Could you check a few things on this model? Use its own coordinates, in mm. A direction names the side the tool comes from. Coordinates: 2 decimals unless noted, no trailing zeros. Order: outer loops, then holes, each group sorted by start corner. A loop starts at its lowest first (then second) coordinate and runs counter-clockwise, first axis right, second up. Notation, with made-up numbers: (76.25, -7) - (134.25, -7) arc R25 cw to (134.25, 28) - close; hole circle Ø10 at (59.25, 4). An arc over 180 degrees is marked (long way). Answer as a JSON object with one key per item and string values. Group by question number.
(1) Imagine slicing it at C-C, the plane z = 3.6. Give the number of separate pieces and of enclosed holes in the cut face, and give its area (3 significant figures).
(2) We'd pull the mould along Y, two halves only. Please class faces 1 (the cylindrical face through (109.745, -109.861, 2.958)), 2 (the flat face through (-2, 2, 6)), 3 (the flat face through (-5, 69, 3)): pulls with the +Y half, pulls with the -Y half, needs draft (parallel to the pull), parting line crosses it, or undercut.
(3) Which directions (+Z, -Z, +X, -X, +Y, -Y) give clear straight access to the entire face, cutting with the end or side of a thin tool? Please do faces 4 (the flat face through (112, -1, 3)), 5 (the cylindrical face through (73.877, 93.387, 2.958)).
(4) Imagine slicing it at A-A, the plane y = -6. Write out the boundary of the cut face in (x, z).
(5) Please list where these lines run through material, in increasing order: probe 1 along Y at (x, z) = (13.5, 2.4); probe 2 along Y at (x, z) = (-97.5, 3.75); probe 3 along X at (y, z) = (104.5, 1.45).
(6) Imagine slicing it at B-B, the plane x = 63. Write out the boundary of the cut face in (y, z), and give its area (3 significant figures).
from build123d import *

# Parameters (mm, degrees)
F0_R     = 1.5
F0_R_2   = 2.25
F1_DEPTH = 6


with BuildPart() as f1:
    # F0 (on Top) → F1 (new body)
    with BuildSketch(Plane.XY):
        with BuildLine():
            Line((104.5, 112), (-104.5, 112))
            ThreePointArc((-104.5, 112), (-109.803301, 109.803301), (-112, 104.5))
            Line((-112, 104.5), (-112, -104.5))
            ThreePointArc((-112, -104.5), (-109.803301, -109.803301), (-104.5, -112))
            Line((-104.5, -112), (104.5, -112))
            ThreePointArc((104.5, -112), (109.803301, -109.803301), (112, -104.5))
            Line((112, -104.5), (112, 104.5))
            ThreePointArc((112, 104.5), (109.803301, 109.803301), (104.5, 112))
        make_face()
        with Locations((-104.5, -104.5)):
            Circle(F0_R, mode=Mode.SUBTRACT)
        with BuildLine():
            Line((-72.615224, -86.757359), (-27.615224, -41.757359))
            ThreePointArc((-27.615224, -41.757359), (-25.668684, -40.456723), (-23.372583, -40))
            Line((-23.372583, -40), (-11, -40))
            ThreePointArc((-11, -40), (-6.757359, -41.757359), (-5, -46))
            Line((-5, -46), (-5, -91))
            ThreePointArc((-5, -91), (-6.757359, -95.242641), (-11, -97))
            Line((-11, -97), (-68.372583, -97))
            ThreePointArc((-68.372583, -97), (-73.91586, -93.296101), (-72.615224, -86.757359))
        make_face(mode=Mode.SUBTRACT)
        with Locations((-97.5, -40)):
            Circle(F0_R_2, mode=Mode.SUBTRACT)
        with BuildLine():
            Line((-89.6, -25), (-85.4, -25))
            ThreePointArc((-85.4, -25), (-83.27868, -25.87868), (-82.4, -28))
            Line((-82.4, -28), (-82.4, -52))
            ThreePointArc((-82.4, -52), (-83.27868, -54.12132), (-85.4, -55))
            Line((-85.4, -55), (-89.6, -55))
            ThreePointArc((-89.6, -55), (-91.72132, -54.12132), (-92.6, -52))
            Line((-92.6, -52), (-92.6, -28))
            ThreePointArc((-92.6, -28), (-91.72132, -25.87868), (-89.6, -25))
        make_face(mode=Mode.SUBTRACT)
        with Locations((-77.5, -40)):
            Circle(F0_R_2, mode=Mode.SUBTRACT)
        with BuildLine():
            ThreePointArc((23.372583, -40), (25.668684, -40.456723), (27.615224, -41.757359))
            Line((27.615224, -41.757359), (72.615224, -86.757359))
            ThreePointArc((72.615224, -86.757359), (73.91586, -93.296101), (68.372583, -97))
            Line((68.372583, -97), (11, -97))
            ThreePointArc((11, -97), (6.757359, -95.242641), (5, -91))
            Line((5, -91), (5, -46))
            ThreePointArc((5, -46), (6.757359, -41.757359), (11, -40))
            Line((11, -40), (23.372583, -40))
        make_face(mode=Mode.SUBTRACT)
        with Locations((104.5, -104.5)):
            Circle(F0_R, mode=Mode.SUBTRACT)
        with Locations((0, -20.5)):
            Circle(F0_R, mode=Mode.SUBTRACT)
        with BuildLine():
            ThreePointArc((97, -68.372583), (93.296101, -73.91586), (86.757359, -72.615224))
            Line((86.757359, -72.615224), (50.242641, -36.100505))
            ThreePointArc((50.242641, -36.100505), (48.942004, -29.561764), (54.485281, -25.857864))
            Line((54.485281, -25.857864), (91, -25.857864))
            ThreePointArc((91, -25.857864), (95.242641, -27.615224), (97, -31.857864))
            Line((97, -31.857864), (97, -68.372583))
        make_face(mode=Mode.SUBTRACT)
        with Locations((-97.5, 40)):
            Circle(F0_R_2, mode=Mode.SUBTRACT)
        with BuildLine():
            ThreePointArc((-82.4, 28), (-83.27868, 25.87868), (-85.4, 25))
            Line((-85.4, 25), (-89.6, 25))
            ThreePointArc((-89.6, 25), (-91.72132, 25.87868), (-92.6, 28))
            Line((-92.6, 28), (-92.6, 52))
            ThreePointArc((-92.6, 52), (-91.72132, 54.12132), (-89.6, 55))
            Line((-89.6, 55), (-85.4, 55))
            ThreePointArc((-85.4, 55), (-83.27868, 54.12132), (-82.4, 52))
            Line((-82.4, 52), (-82.4, 28))
        make_face(mode=Mode.SUBTRACT)
        with Locations((-77.5, 40)):
            Circle(F0_R_2, mode=Mode.SUBTRACT)
        with Locations((-104.5, 104.5)):
            Circle(F0_R, mode=Mode.SUBTRACT)
        with BuildLine():
            ThreePointArc((-11, 97), (-6.757359, 95.242641), (-5, 91))
            Line((-5, 91), (-5, 46))
            ThreePointArc((-5, 46), (-6.757359, 41.757359), (-11, 40))
            Line((-11, 40), (-23.372583, 40))
            ThreePointArc((-23.372583, 40), (-25.668684, 40.456723), (-27.615224, 41.757359))
            Line((-27.615224, 41.757359), (-72.615224, 86.757359))
            ThreePointArc((-72.615224, 86.757359), (-73.91586, 93.296101), (-68.372583, 97))
            Line((-68.372583, 97), (-11, 97))
        make_face(mode=Mode.SUBTRACT)
        with Locations((0, 20.5)):
            Circle(F0_R, mode=Mode.SUBTRACT)
        with Locations((77.5, 0)):
            Circle(F0_R_2, mode=Mode.SUBTRACT)
        with BuildLine():
            Line((85.4, 15), (89.6, 15))
            ThreePointArc((89.6, 15), (91.72132, 14.12132), (92.6, 12))
            Line((92.6, 12), (92.6, -12))
            ThreePointArc((92.6, -12), (91.72132, -14.12132), (89.6, -15))
            Line((89.6, -15), (85.4, -15))
            ThreePointArc((85.4, -15), (83.27868, -14.12132), (82.4, -12))
            Line((82.4, -12), (82.4, 12))
            ThreePointArc((82.4, 12), (83.27868, 14.12132), (85.4, 15))
        make_face(mode=Mode.SUBTRACT)
        with Locations((97.5, 0)):
            Circle(F0_R_2, mode=Mode.SUBTRACT)
        with BuildLine():
            ThreePointArc((54.485281, 25.857864), (48.942004, 29.561764), (50.242641, 36.100505))
            Line((50.242641, 36.100505), (86.757359, 72.615224))
            ThreePointArc((86.757359, 72.615224), (93.296101, 73.91586), (97, 68.372583))
            Line((97, 68.372583), (97, 31.857864))
            ThreePointArc((97, 31.857864), (95.242641, 27.615224), (91, 25.857864))
            Line((91, 25.857864), (54.485281, 25.857864))
        make_face(mode=Mode.SUBTRACT)
        with BuildLine():
            Line((5, 46), (5, 91))
            ThreePointArc((5, 91), (6.757359, 95.242641), (11, 97))
            Line((11, 97), (68.372583, 97))
            ThreePointArc((68.372583, 97), (73.91586, 93.296101), (72.615224, 86.757359))
            Line((72.615224, 86.757359), (27.615224, 41.757359))
            ThreePointArc((27.615224, 41.757359), (25.668684, 40.456723), (23.372583, 40))
            Line((23.372583, 40), (11, 40))
            ThreePointArc((11, 40), (6.757359, 41.757359), (5, 46))
        make_face(mode=Mode.SUBTRACT)
        with Locations((104.5, 104.5)):
            Circle(F0_R, mode=Mode.SUBTRACT)
    extrude(amount=F1_DEPTH)


solid = f1.part
Result set:
{
 "1": {"separate pieces": "1", "enclosed holes": "21", "area": "35,000 mm^2"},
 "2": {"face 1": "pulls with the -Y half", "face 2": "needs draft", "face 3": "undercut"},
 "3": {"face 4": "+Z, -Z, +X, +Y, -Y", "face 5": "+Z, -Z"},
 "4": {"outline": "(-112, 0) - (82.4, 0) - (82.4, 6) - (-112, 6) - close; (92.6, 0) - (112, 0) - (112, 6) - (92.6, 6) - close"},
 "5": {"probe 1": "y = -112 to -97, -40 to 40, 97 to 112", "probe 2": "y = -112 to -42.25, -37.75 to 37.75, 42.25 to 112", "probe 3": "x = -112 to -106, -103 to 103, 106 to 112"},
 "6": {"outline": "(-112, 0) - (-97, 0) - (-97, 6) - (-112, 6) - close; (-77.14, 0) - (-48.86, 0) - (-48.86, 6) - (-77.14, 6) - close; (-25.86, 0) - (25.86, 0) - (25.86, 6) - (-25.86, 6) - close; (48.86, 0) - (77.14, 0) - (77.14, 6) - (48.86, 6) - close; (97, 0) - (112, 0) - (112, 6) - (97, 6) - close", "area": "830 mm^2"}
}
